```python
from build123d import *

# Parameters (mm, degrees)
SKETCH1_W                  = 40
SKETCH1_H                  = 22
BOSS_EXTRUDE1_DEPTH        = 11
SKETCH2_W                  = 40
SKETCH2_H                  = 22
SKETCH2_R                  = 4.25
BOSS_EXTRUDE2_DEPTH        = 7
SKETCH3_W                  = 24.5
SKETCH3_H                  = 15.5
CUT_EXTRUDE1_DEPTH         = 7.75
FILLET1_R                  = 7.75
SKETCH4_R                  = 5
CUT_EXTRUDE2_DEPTH         = 36.805900352
SKETCH5_W                  = 8
SKETCH5_H                  = 8
SKETCH5_R                  = 1.905800151
BOSS_EXTRUDE3_DEPTH        = 6
CUT_EXTRUDE3_START         = -3
SKETCH6_R                  = 3
SKETCH6_R_2                = 1.905800151
CUT_EXTRUDE3_DEPTH         = 3
SKETCH7_W                  = 16
SKETCH7_H                  = 16.5
BOSS_EXTRUDE5_DEPTH        = 28
MIRROR14_COPY_1_SKETCH_W   = 8
MIRROR14_COPY_1_SKETCH_H   = 8
MIRROR14_COPY_1_SKETCH_R   = 1.905800151
MIRROR14_COPY_1_DEPTH      = 6
MIRROR14_START             = -3
MIRROR14_COPY_2_SKETCH_R   = 3
MIRROR14_COPY_2_SKETCH_R_2 = 1.905800151
MIRROR14_COPY_2_DEPTH      = 3
FILLET1_OF_MIRROR14_R      = 7.75
SKETCH9_W                  = 28
SKETCH9_H                  = 3
BOSS_EXTRUDE6_DEPTH        = 18
CUT_EXTRUDE4_DEPTH         = 10
CUT_EXTRUDE5_DEPTH         = 74.288812243
CUT_EXTRUDE5_DEPTH_BACK    = 74.288812243
SKETCH11_R                 = 1.75
CUT_EXTRUDE6_DEPTH         = 76.121568141
CUT_EXTRUDE6_DEPTH_BACK    = 76.121568141
SKETCH12_R                 = 1.75
FILLET2_R                  = 2
CUT_EXTRUDE12_START        = -3
SKETCH17_R                 = 1.75
CUT_EXTRUDE12_DEPTH        = 3
CUT_EXTRUDE13_DEPTH        = 74.097537578
CUT_EXTRUDE13_DEPTH_BACK   = 74.097537578
SKETCH18_W                 = 18
SKETCH18_H                 = 5
FILLET3_R                  = 2.5
CUT_EXTRUDE14_DEPTH        = 74.710582687
CUT_EXTRUDE15_START        = -10
SKETCH21_R                 = 1.75
CUT_EXTRUDE15_DEPTH        = 10
SKETCH20_W                 = 36.163748027
SKETCH20_H                 = 4
CUT_EXTRUDE16_DEPTH        = 13.5
SKETCH22_W                 = 6.75
SKETCH22_H                 = 13.5
CUT_EXTRUDE18_DEPTH        = 8
SKETCH23_R                 = 4.25
BOSS_EXTRUDE8_DEPTH        = 1


with BuildPart() as part:
    # Sketch1 → Boss-Extrude1 (new body)
    with BuildSketch(Plane(origin=(0, 0, 0), x_dir=(1, 0, 0), z_dir=(0, 1, 0))):
        Rectangle(SKETCH1_W, SKETCH1_H)
    boss_extrude1 = extrude(amount=BOSS_EXTRUDE1_DEPTH)

    # Sketch2 → Boss-Extrude2 (add)
    with BuildSketch(Plane(origin=(0, 0, 0), x_dir=(1, 0, 0), z_dir=(0, 1, 0))):
        Rectangle(SKETCH2_W, SKETCH2_H)
        with Locations(Location((0, 0, 0), (0, 0, 270))):
            Circle(SKETCH2_R, mode=Mode.SUBTRACT)
    boss_extrude2 = extrude(amount=-BOSS_EXTRUDE2_DEPTH)

    # Sketch3 → Cut-Extrude1 (cut)
    with BuildSketch(Plane(origin=(0, 11, 0), x_dir=(1, 0, 0), z_dir=(0, 1, 0))):
        Rectangle(SKETCH3_W, SKETCH3_H)
    cut_extrude1 = extrude(amount=-CUT_EXTRUDE1_DEPTH, mode=Mode.SUBTRACT)

    # Fillet1
    fillet1_edges = [part.edges().sort_by_distance(p)[0] for p in [
        (0, 3.25, 7.75),
        (0, 3.25, -7.75),
    ]]
    fillet(fillet1_edges, radius=FILLET1_R - 0.0001)  # a hair under: the kernel refuses the full size

    # Sketch4 → Cut-Extrude2 (cut, symmetric)
    with BuildSketch(Plane(origin=(-12.25, 0, 0), x_dir=(0, 0, -1), z_dir=(1, 0, 0))):
        with Locations((0, 11)):
            Circle(SKETCH4_R)
    cut_extrude2 = extrude(amount=CUT_EXTRUDE2_DEPTH, both=True, mode=Mode.SUBTRACT)

    # Sketch5 → Boss-Extrude3 (add)
    with BuildSketch(Plane(origin=(0, 11, 0), x_dir=(1, 0, 0), z_dir=(0, 1, 0))):
        with Locations((16, -15)):
            Rectangle(SKETCH5_W, SKETCH5_H)
        with Locations(Location((16, -15, 0), (0, 0, 270))):
            Circle(SKETCH5_R, mode=Mode.SUBTRACT)
    boss_extrude3 = extrude(amount=-BOSS_EXTRUDE3_DEPTH)

    # Sketch6 → Cut-Extrude3 (cut)
    with BuildSketch(Plane.XZ.offset(-5).offset(CUT_EXTRUDE3_START)):
        with Locations(Location((16, 15, 0), (0, 0, 270))):
            Circle(SKETCH6_R)
        with Locations(Location((16, 15, 0), (0, 0, 90))):
            Circle(SKETCH6_R_2, mode=Mode.SUBTRACT)
    cut_extrude3 = extrude(amount=CUT_EXTRUDE3_DEPTH, mode=Mode.SUBTRACT)

    # Mirror8: Boss-Extrude3, Cut-Extrude3 across plane
    add(boss_extrude3.mirror(Plane(origin=(0, 0, 0), x_dir=(0, 0, 1), z_dir=(1, 0, 0))))
    add(cut_extrude3.mirror(Plane(origin=(0, 0, 0), x_dir=(0, 0, 1), z_dir=(1, 0, 0))), mode=Mode.SUBTRACT)

    # Sketch7 → Boss-Extrude5 (add)
    with BuildSketch(Plane(origin=(0, 0, -11), x_dir=(-1, 0, 0), z_dir=(0, 0, -1))):
        with Locations((-12, 9.25)):
            Rectangle(SKETCH7_W, SKETCH7_H)
    extrude(amount=BOSS_EXTRUDE5_DEPTH)

    # Mirror14: Boss-Extrude1, Boss-Extrude2, Cut-Extrude1, Cut-Extrude2, Boss-Extrude3, Cut-Extrude3 across plane
    add(boss_extrude1.mirror(Plane.XY.offset(-25)))
    add(boss_extrude2.mirror(Plane.XY.offset(-25)))
    add(cut_extrude1.mirror(Plane.XY.offset(-25)), mode=Mode.SUBTRACT)
    add(cut_extrude2.mirror(Plane.XY.offset(-25)), mode=Mode.SUBTRACT)
    add(boss_extrude3.mirror(Plane.XY.offset(-25)))
    add(cut_extrude3.mirror(Plane.XY.offset(-25)), mode=Mode.SUBTRACT)

    # Mirror14 copy 1 sketch → Mirror14 copy 1 (add)
    with BuildSketch(Plane(origin=(0, 11, -50), x_dir=(-1, 0, 0), z_dir=(0, 1, 0))):
        with Locations((16, -15)):
            Rectangle(MIRROR14_COPY_1_SKETCH_W, MIRROR14_COPY_1_SKETCH_H)
        with Locations(Location((16, -15, 0), (0, 0, 270))):
            Circle(MIRROR14_COPY_1_SKETCH_R, mode=Mode.SUBTRACT)
    extrude(amount=-MIRROR14_COPY_1_DEPTH)

    # Mirror14 copy 2 sketch → Mirror14 copy 2 (cut)
    with BuildSketch(Plane(origin=(0, 5, -50), x_dir=(-1, 0, 0), z_dir=(0, -1, 0)).offset(MIRROR14_START)):
        with Locations(Location((16, 15, 0), (0, 0, 270))):
            Circle(MIRROR14_COPY_2_SKETCH_R)
        with Locations(Location((16, 15, 0), (0, 0, 90))):
            Circle(MIRROR14_COPY_2_SKETCH_R_2, mode=Mode.SUBTRACT)
    extrude(amount=MIRROR14_COPY_2_DEPTH, mode=Mode.SUBTRACT)

    # Fillet1 of Mirror14
    fillet1_of_mirror14_edges = [part.edges().sort_by_distance(p)[0] for p in [
        (0, 3.25, -57.75),
        (0, 3.25, -42.25),
    ]]
    fillet(fillet1_of_mirror14_edges, radius=FILLET1_OF_MIRROR14_R - 0.0001)  # a hair under: the kernel refuses the full size

    # Sketch9 → Boss-Extrude6 (add)
    with BuildSketch(Plane.ZY.offset(-4)):
        with Locations((-25, 2.5)):
            Rectangle(SKETCH9_W, SKETCH9_H)
    extrude(amount=BOSS_EXTRUDE6_DEPTH)

    # Sketch10 → Cut-Extrude4 (cut)
    with BuildSketch(Plane(origin=(0, 17.5, 0), x_dir=(1, 0, 0), z_dir=(0, 1, 0))):
        with BuildLine():
            Line((9, 26.25), (9, 23.75))
            Line((9, 23.75), (11.727178029, 23.75))
            ThreePointArc((11.727178029, 23.75), (11.931001031, 24.360286817), (12, 25))
            ThreePointArc((12, 25), (11.931001031, 25.639713183), (11.727178029, 26.25))
            Line((11.727178029, 26.25), (9, 26.25))
        make_face()
        with BuildLine():
            Line((11.727178029, 23.75), (9, 23.75))
            Line((9, 23.75), (9, 26.25))
            Line((9, 26.25), (11.727178029, 26.25))
            ThreePointArc((11.727178029, 26.25), (6, 25), (11.727178029, 23.75))
        make_face()
        with BuildLine():
            ThreePointArc((12, 25), (11.931001031, 24.360286817), (11.727178029, 23.75))
            Line((11.727178029, 23.75), (20, 23.75))
            Line((20, 23.75), (20, 26.25))
            Line((20, 26.25), (11.727178029, 26.25))
            ThreePointArc((11.727178029, 26.25), (11.931001031, 25.639713183), (12, 25))
        make_face()
    extrude(amount=-CUT_EXTRUDE4_DEPTH, mode=Mode.SUBTRACT)

    # Sketch11 → Cut-Extrude5 (cut, two sides: drawn at the far end of the back side and taken through both)
    with BuildSketch(Plane(origin=(0, 7.5, 0), x_dir=(1, 0, 0), z_dir=(0, 1, 0)).offset(-CUT_EXTRUDE5_DEPTH_BACK)):
        with Locations(Location((9, 25, 0), (0, 0, 270))):
            Circle(SKETCH11_R)
    extrude(amount=CUT_EXTRUDE5_DEPTH + CUT_EXTRUDE5_DEPTH_BACK, mode=Mode.SUBTRACT)

    # Sketch12 → Cut-Extrude6 (cut, two sides: drawn at the far end of the back side and taken through both)
    with BuildSketch(Plane.ZY.offset(-4).offset(-CUT_EXTRUDE6_DEPTH_BACK)):
        with Locations((-31, 11)):
            Circle(SKETCH12_R)
    extrude(amount=CUT_EXTRUDE6_DEPTH + CUT_EXTRUDE6_DEPTH_BACK, mode=Mode.SUBTRACT)

    # Fillet2
    fillet2_edges = [part.edges().sort_by_distance(p)[0] for p in [
        (11.727178029, 12.5, -23.75),
        (11.727178029, 12.5, -26.25),
    ]]
    fillet(fillet2_edges, radius=FILLET2_R)

    # Sketch17 → Cut-Extrude12 (cut)
    with BuildSketch(Plane.XZ.offset(-1).offset(CUT_EXTRUDE12_START)):
        Polygon((12.175426481, -25), (10.58771324, -22.25), (7.41228676, -22.25), (5.824573519, -25), (7.41228676, -27.75), (10.58771324, -27.75), align=None)
        with Locations(Location((9, -25, 0), (0, 0, 90))):
            Circle(SKETCH17_R, mode=Mode.SUBTRACT)
    extrude(amount=CUT_EXTRUDE12_DEPTH, mode=Mode.SUBTRACT)

    # Sketch18 → Cut-Extrude13 (cut, two sides: drawn at the far end of the back side and taken through both)
    with BuildSketch(Plane(origin=(0, 4, 0), x_dir=(1, 0, 0), z_dir=(0, 1, 0)).offset(-CUT_EXTRUDE13_DEPTH_BACK)):
        with Locations((-5, 25)):
            Rectangle(SKETCH18_W, SKETCH18_H)
    extrude(amount=CUT_EXTRUDE13_DEPTH + CUT_EXTRUDE13_DEPTH_BACK, mode=Mode.SUBTRACT)

    # Fillet3
    fillet3_edges = [part.edges().sort_by_distance(p)[0] for p in [
        (4, 2.5, -27.5),
        (4, 2.5, -22.5),
    ]]
    fillet(fillet3_edges, radius=FILLET3_R - 0.0001)  # a hair under: the kernel refuses the full size

    # Sketch19 → Cut-Extrude14 (cut, through all)
    with BuildSketch(Plane.XZ.offset(-1)):
        Polygon((20, -61), (20, -39), (-14, -39), (-20, -39), (-20, -61), align=None)
    extrude(amount=CUT_EXTRUDE14_DEPTH, mode=Mode.SUBTRACT)

    # Sketch21 → Cut-Extrude15 (cut)
    with BuildSketch(Plane(origin=(20, 0, 0), x_dir=(0, 0, -1), z_dir=(1, 0, 0)).offset(CUT_EXTRUDE15_START)):
        Polygon((31, 14.175426481), (28.25, 12.58771324), (28.25, 9.41228676), (31, 7.824573519), (33.75, 9.41228676), (33.75, 12.58771324), align=None)
        with Locations((31, 11)):
            Circle(SKETCH21_R, mode=Mode.SUBTRACT)
    extrude(amount=CUT_EXTRUDE15_DEPTH, mode=Mode.SUBTRACT)

    # Sketch20 → Cut-Extrude16 (cut)
    with BuildSketch(Plane(origin=(0, 17.5, 0), x_dir=(1, 0, 0), z_dir=(0, 1, 0))):
        with Locations((22.081874014, 37)):
            Rectangle(SKETCH20_W, SKETCH20_H)
    extrude(amount=-CUT_EXTRUDE16_DEPTH, mode=Mode.SUBTRACT)

    # Sketch22 → Cut-Extrude18 (cut)
    with BuildSketch(Plane(origin=(20, 0, 0), x_dir=(0, 0, -1), z_dir=(1, 0, 0))):
        with Locations((31.625, 10.75)):
            Rectangle(SKETCH22_W, SKETCH22_H)
    extrude(amount=-CUT_EXTRUDE18_DEPTH, mode=Mode.SUBTRACT)

    # Sketch23 → Boss-Extrude8 (add)
    with BuildSketch(Plane.XZ):
        with Locations(Location((0, 0, 0), (0, 0, 90))):
            Circle(SKETCH23_R)
    extrude(amount=BOSS_EXTRUDE8_DEPTH)


solid = part.part
```
Design review of the part built by this model. Coordinates are the model's own, in mm. A direction names the side the tool comes from. Give positions to 0.01 mm unless a question says otherwise; leave off trailing zeros. Order: outer loops, then holes, each group sorted by start corner. A loop starts at its lowest first (then second) coordinate and runs counter-clockwise, first axis right, second up. Notation, with made-up numbers: (-1, -9) - (49, -9) arc R22 cw to (49, 11) - close; hole circle Ø2 at (3.25, 46.25). An arc over 180 degrees is marked (long way). Use a Markdown table: item, result. Add a question column.
(1) Wall thickness on probe 1 along X at (y, z) = (9.4, 15); probe 2 along X at (y, z) = (7.2, 15); probe 3 along Z at (x, y) = (-2, 8.5): over which ranges is each line inside the solid? List them lowest first. Write a range as [from, to].
(2) Machinability: for faces 4 (the face through (10.986, 13.37, -32.394)), 5 (the face through (0.17, 5.58, -44.46)), 6 (the face through (3, 3, -23)), 7 (the face through (4.214, -3.958, -0.553)), which of the approach directions +Z, -Z, +X, -X, +Y, -Y give a long, thin tool a straight path to every point of the face, cutting with its end or side? Answer none if there is none.
(3) Mouldability with a two-part tool opening along Z and no side actions: class faces 1 (the face through (0, 0, 11)), 2 (the face through (10.986, 8.63, -29.606)), 3 (the face through (-12, 8, -65)) as +Z half, -Z half, draft (parallel to the pull), parting line (faces both ways), or undercut.
(4) Clearance check with flat-ended pins moving along their axes: P1, Ø1.8, axis at x = 16, z = 16.5, coming from the -Y side; P2, Ø6, axis at x = 7.5, z = 2.5, coming from the +Y side; P3, Ø7, axis at x = -3, z = -28.5, coming from the +Y side. State where each tip first meets the part, or that it passes through.
(5) Add section C-C on z = -65. Give the boundary of the cut face in (x, y), then the cut area to 3 significant figures.
(6) Add section B-B on x = -16. Give the number of separate pieces and of enclosed holes in the cut face, then the cut area to 3 significant figures.
Report:
| question | item | result |
|---|---|---|
| 1 | probe 1 | x = [-20, -17.91], [-14.09, -12], [12, 14.09], [17.91, 20] |
| 1 | probe 2 | x = [-20, -19], [-13, -12], [12, 13], [19, 20] |
| 1 | probe 3 | z = [-61, -57.34], [-42.66, -39], [-11, -7.34], [7.34, 11] |
| 2 | face 4 | +X |
| 2 | face 5 | +Y |
| 2 | face 6 | -X, +Y, -Y |
| 2 | face 7 | -Y |
| 3 | face 1 | +Z half |
| 3 | face 2 | undercut |
| 3 | face 3 | draft |
| 4 | P1 | stops at y = 8 |
| 4 | P2 | stops at y = 5.54 |
| 4 | P3 | stops at y = 4 |
| 5 | outline | (-20, 5) - (-19, 5) - (-19, 8) - (-17.91, 8) - (-17.91, 11) - (-20, 11) - close; (-14.09, 8) - (-13, 8) - (-13, 5) - (-12, 5) - (-12, 11) - (-14.09, 11) - close; (12, 5) - (13, 5) - (13, 8) - (14.09, 8) - (14.09, 11) - (12, 11) - close; (17.91, 8) - (19, 8) - (19, 5) - (20, 5) - (20, 11) - (17.91, 11) - close |
| 5 | area | 37.1 mm² |
| 6 | separate pieces | 4 |
| 6 | enclosed holes | 0 |
| 6 | area | 575 mm² |
